Read the model definition and answer for the solid it produces. Units are mm, in the model's axes. A direction names the side the tool comes from. Coordinates: 2 decimals unless noted, no trailing zeros. Write each loop counter-clockwise with the first axis right and the second up, starting at its lowest first coordinate (ties: lowest second). Pieces come first, ordered by that corner, then holes. Notation, with made-up numbers: (81, 52.25) - (105, 52.25) arc R32 cw to (105, 83.25) - close; hole circle Ø2 at (10, 51.5). An arc over 180 degrees is marked (long way). Return JSON: item names as keys, results as strings.
```python
from build123d import *

# Parameters (mm, degrees)
SKETCH1_R           = 21.5
SKETCH1_R_2         = 18.38
BOSS_EXTRUDE1_DEPTH = 29.5
SKETCH3_R           = 21.5
BOSS_EXTRUDE2_DEPTH = 1
SKETCH4_R           = 2
SKETCH4_R_2         = 0.75
BOSS_EXTRUDE3_DEPTH = 3.8
SKETCH5_OUTSIDE_W   = 58.518
SKETCH5_OUTSIDE_H   = 58.518
SKETCH5_OUTSIDE_R   = 20
CUT_EXTRUDE1_DEPTH  = 3.5
CUT_EXTRUDE2_REACH  = 37.488
CIRPATTERN1_COUNT   = 6


with BuildPart() as part:
    # Sketch1 → Boss-Extrude1 (new body)
    with BuildSketch(Plane(origin=(0, 0, 0), x_dir=(1, 0, 0), z_dir=(0, 1, 0))):
        with Locations(Location((0, 0, 0), (0, 0, 270))):
            Circle(SKETCH1_R)
        with Locations(Location((0, 0, 0), (0, 0, 270))):
            Circle(SKETCH1_R_2, mode=Mode.SUBTRACT)
    extrude(amount=BOSS_EXTRUDE1_DEPTH)

    # Sketch3 → Boss-Extrude2 (add)
    with BuildSketch(Plane(origin=(0, 11.2, 0), x_dir=(-1, 0, 0), z_dir=(0, -1, 0))):
        with Locations(Location((0, 0, 0), (0, 0, 270))):
            Circle(SKETCH3_R)
    extrude(amount=-BOSS_EXTRUDE2_DEPTH)

    # Sketch4 → Boss-Extrude3 (add)
    with BuildSketch(Plane(origin=(0, 11.2, 0), x_dir=(-1, 0, 0), z_dir=(0, -1, 0))):
        with Locations(Location((0, 0, 0), (0, 0, 270))):
            Circle(SKETCH4_R)
        with Locations(Location((0, 0, 0), (0, 0, 270))):
            Circle(SKETCH4_R_2, mode=Mode.SUBTRACT)
    extrude(amount=BOSS_EXTRUDE3_DEPTH)

    # Sketch5 outside → Cut-Extrude1 (cut)
    with BuildSketch(Plane(origin=(0, 0, 0), x_dir=(1, 0, 0), z_dir=(0, 1, 0))):
        Rectangle(SKETCH5_OUTSIDE_W, SKETCH5_OUTSIDE_H)
        with Locations(Location((0, 0, 0), (0, 0, 270))):
            Circle(SKETCH5_OUTSIDE_R, mode=Mode.SUBTRACT)
    extrude(amount=CUT_EXTRUDE1_DEPTH, mode=Mode.SUBTRACT)

    # Sketch6 → Cut-Extrude2 (cut, up to next)
    with BuildSketch(Plane(origin=(0, 11.2, 0), x_dir=(-1, 0, 0), z_dir=(0, -1, 0)), mode=Mode.PRIVATE) as cut_extrude2_sk1:
        with BuildLine():
            Line((1.311528297, -4.358954791), (1.311528297, -15.245444515))
            ThreePointArc((1.311528297, -15.245444515), (1.659572625, -16.003701596), (2.461435901, -16.234144525))
            ThreePointArc((2.461435901, -16.234144525), (8.209843408, -14.219865905), (12.828463617, -10.248738282))
            ThreePointArc((12.828463617, -10.248738282), (13.029825824, -9.439082851), (12.547178093, -8.75853908))
            Line((12.547178093, -8.75853908), (3.119201435, -3.315294219))
            ThreePointArc((3.119201435, -3.315294219), (2.601197124, -3.181481713), (2.088346263, -3.333857065))
            ThreePointArc((2.088346263, -3.333857065), (1.966964225, -3.406881974), (1.843031779, -3.475489448))
            ThreePointArc((1.843031779, -3.475489448), (1.454645424, -3.843443646), (1.311528297, -4.358954791))
        make_face()
    cut_extrude2_tool1 = extrude(cut_extrude2_sk1.sketch, amount=-CUT_EXTRUDE2_REACH, mode=Mode.PRIVATE) & part.part
    cut_extrude2 = cut_extrude2_tool1.solids().sort_by_distance((-5.765973, 11.2, 9.986958))[0]
    add(cut_extrude2, mode=Mode.SUBTRACT)

    # CirPattern1: Cut-Extrude2 ×6 about axis
    cirpattern1_axis = Axis((0, 0, 0), (0, 1, 0))
    for i in range(1, CIRPATTERN1_COUNT):
        add(cut_extrude2.rotate(cirpattern1_axis, i * 360 / CIRPATTERN1_COUNT), mode=Mode.SUBTRACT)


solid = part.part
```
(1) A cutting plane is placed at A-A (y = 9.75). Determine the outline of the cut face in (x, z).
Answer:
{"outline": "circle Ø43 at (0, 0); circle Ø4 at (0, 0); hole circle Ø36.76 at (0, 0); hole circle Ø1.5 at (0, 0)"}
(2) Which of the six approach directions +Z, -Z, +X, -X, +Y, -Y give full straight-line access (tool end or side, diameter ignored) to faces 1 (the face through (7.899, 11.693, -6.075)), 2 (the face through (0, 12.2, 0)), 3 (the face through (2, 9, 0))?
Answer:
{"face 1": "+Y, -Y", "face 2": "+Y", "face 3": "-Y"}
(3) Determine the mould class of faces 4 (the face through (-19.524, 1.726, -4.336)), 5 (the face through (10, 29.5, 16)), 6 (the face through (0, 11.2, 0)) for opening direction Z: +Z half, -Z half, draft (parallel to the pull), parting line (faces both ways), or undercut.
Answer:
{"face 4": "parting line", "face 5": "draft", "face 6": "undercut"}
(4) Flat-ended cylindrical pins translate along their axes: P1, Ø12, axis at y = 18, z = 7, coming from the +X side; P2, Ø0.5, axis at y = 12, z = -12.5, coming from the +X side; P3, Ø12, axis at y = 6, z = 5, coming from the -X side. Find the tip coordinate at first contact, or state that the pin passes through.
Answer:
{"P1": "x = 21.48", "P2": "x = 17.67", "P3": "x = -21.5"}
(5) Straight lines are drawn through the part: line 1 (X direction, y = 10.2, z = 0); line 2 (X direction, y = 3.75, z = 0); line 3 (Y direction, x = 0, z = -1.5). For each, find the intervals that lie inside material, in ascending order. Write a range as from..to.
Answer:
{"line 1": "-21.5..-18.38, -2..-0.75, 0.75..2, 18.38..21.5", "line 2": "-21.5..-18.38, 18.38..21.5", "line 3": "7.4..12.2"}
(6) A cutting plane is placed at B-B (x = 5). Determine the outline of the cut face in (y, z).
Answer:
{"outline": "(0, -19.36) - (3.5, -19.36) - (3.5, -20.91) - (29.5, -20.91) - (29.5, -17.69) - (12.2, -17.69) - (12.2, -15.64) - (11.2, -15.64) - (11.2, -17.69) - (0, -17.69) - close; (0, 17.69) - (11.2, 17.69) - (11.2, 15.64) - (12.2, 15.64) - (12.2, 17.69) - (29.5, 17.69) - (29.5, 20.91) - (3.5, 20.91) - (3.5, 19.36) - (0, 19.36) - close; (11.2, -4.4) - (12.2, -4.4) - (12.2, -1.37) - (11.2, -1.37) - close; (11.2, 1.37) - (12.2, 1.37) - (12.2, 4.4) - (11.2, 4.4) - close"}
(7) A cutting plane is placed at C-C (z = 5). State how many separate pieces and enclosed holes the cut face has, and give its area (3 significant figures).
Answer:
{"separate pieces": "5", "enclosed holes": "0", "area": "197 mm²"}
(8) A cutting plane is placed at D-D (x = 0). Determine the outline of the cut face in (y, z), and give its area (3 significant figures).
Answer:
{"outline": "(0, -20) - (3.5, -20) - (3.5, -21.5) - (29.5, -21.5) - (29.5, -18.38) - (12.2, -18.38) - (12.2, 18.38) - (29.5, 18.38) - (29.5, 21.5) - (3.5, 21.5) - (3.5, 20) - (0, 20) - (0, 18.38) - (11.2, 18.38) - (11.2, 2) - (7.4, 2) - (7.4, 0.75) - (11.2, 0.75) - (11.2, -0.75) - (7.4, -0.75) - (7.4, -2) - (11.2, -2) - (11.2, -18.38) - (0, -18.38) - close", "area": "220 mm²"}
